Here's how the part is built. I have some questions about the finished solid (model axes, mm). Face numbers are marked on the shaded views. A direction names the side the tool comes from. Give positions to 0.01 mm unless a question says otherwise; leave off trailing zeros. Order: outer loops, then holes, each group sorted by start corner. A loop starts at its lowest first (then second) coordinate and runs counter-clockwise, first axis right, second up. Notation, with made-up numbers: (57, -30.75) -> (96, -30.75) arc R8 cw to (96, -17.75) -> close; hole circle Ø10 at (33, 34.25). An arc over 180 degrees is marked (long way). Write each question's results on one line, items separated by ' | '. Start each with the question number.
Q1. Imagine slicing it at A-A, the plane x = 0. Please give me the cut outline in (y, z), then the cut area to 3 significant figures.
Q2. For the marked faces 1, 2 and 3, which set-ups out of +Z, -Z, +X, -X, +Y, -Y let a thin tool reach every point of the face, with its end or its side?
Q3. I'm going to push flat-ended pins straight in: pin 1 (3.5 mm diameter, centred on x = -23, z = 51.5, fed in from +Y); pin 2 (8 mm diameter, centred on x = -13, z = 67, fed in from +Y); pin 3 (6 mm diameter, centred on x = 0.5, z = 38.5, fed in from +Y); pin 4 (1 mm diameter, centred on x = 7, y = 8, fed in from +Z). Where does each tip first touch, or does it pass through?
Q4. Imagine slicing it at D-D, the plane x = 23. Please give me the cut outline in (y, z).
Q5. Thinking about a two-plate mould opening in Y: for the marked faces 4, 5 and 6, which applies, pulls with the +Y half, pulls with the -Y half, needs draft (parallel to the pull), parting line crosses it, or undercut?
Q6. Imagine slicing it at C-C, the plane y = 29. Please give me the cut outline in (x, z).
Q7. I need wall thicknesses on line 1 along Y through (x, z) = (0, 51.5); line 2 along X through (y, z) = (27, 60.5); line 3 along Y through (x, z) = (-4, 73.5). Which ranges of each line are inside material? Lowest first, please. Write a range as [from, to].
Q8. Imagine slicing it at B-B, the plane z = 25.5. Please give me the cut outline in (x, y), then the cut area to 3 significant figures.
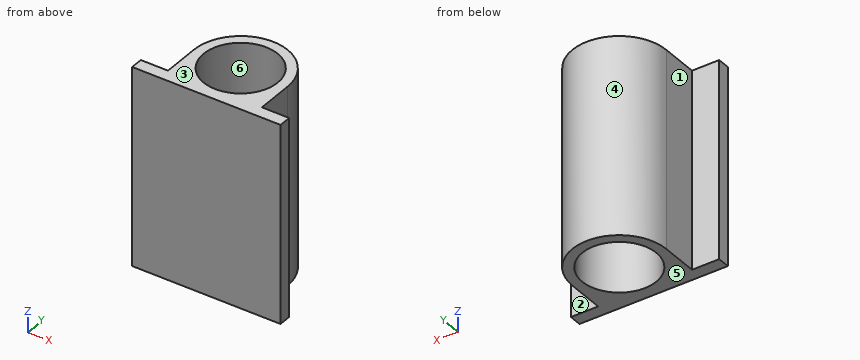
```python
from build123d import *

# Parameters (mm, degrees)
SKETCH_R  = 15
PAD_DEPTH = 80


with BuildPart() as part:
    # Sketch → Pad (new body)
    with BuildSketch(Plane.XY):
        with BuildLine():
            Line((30, 5), (30, 0))
            Line((30, 0), (-30, 0))
            Line((-30, 0), (-30, 5))
            Line((-30, 5), (-19, 5))
            Line((-19, 20), (-19, 5))
            ThreePointArc((19, 20), (0, 39), (-19, 20))
            Line((19, 20), (19, 5))
            Line((19, 5), (30, 5))
        make_face()
        with Locations((0, 20)):
            Circle(SKETCH_R, mode=Mode.SUBTRACT)
    extrude(amount=PAD_DEPTH)


solid = part.part
```
Geometry check:
1) outline: (0, 0) -> (5, 0) -> (5, 80) -> (0, 80) -> close; (35, 0) -> (39, 0) -> (39, 80) -> (35, 80) -> close | area: 720 mm²
2) face 1: +Z, -Z, -X, +Y | face 2: +Z, -Z, +X, +Y | face 3: +Z, +X, -X, +Y, -Y
3) pin 1: y = 5 | pin 2: y = 36.73 | pin 3: y = 39 | pin 4: through
4) outline: (0, 0) -> (5, 0) -> (5, 80) -> (0, 80) -> close
5) face 4: pulls with the +Y half | face 5: needs draft | face 6: undercut
6) outline: (-16.73, 0) -> (-12, 0) -> (-12, 80) -> (-16.73, 80) -> close; (12, 0) -> (16.73, 0) -> (16.73, 80) -> (12, 80) -> close
7) line 1: [0, 5], [35, 39] | line 2: [-17.66, -13.27], [13.27, 17.66] | line 3: [0, 5.54], [34.46, 38.57]
8) outline: (-30, 0) -> (30, 0) -> (30, 5) -> (19, 5) -> (19, 20) arc R19 ccw to (-19, 20) -> (-19, 5) -> (-30, 5) -> close; hole circle Ø30 at (0, 20) | area: 730 mm²
